Model file for the job. Use its own axes, mm. Face numbers are marked on the shaded views. A direction names the side the tool comes from. Round coordinates to 2 decimals unless told otherwise and drop trailing zeros. Loops run counter-clockwise (first coordinate to the right, second up) from the corner with the lowest first, then second, coordinate; pieces in that order, holes last.
from build123d import *

# Parameters (mm, degrees)
BOSS_EXTRUDE1_DEPTH = 12
SKETCH2_W           = 4
SKETCH2_H           = 1.5
BOSS_EXTRUDE2_DEPTH = 10
CUT_EXTRUDE1_DEPTH  = 2.5
BOSS_EXTRUDE4_DEPTH = 6
SKETCH6_R           = 2.275
BOSS_EXTRUDE5_DEPTH = 3.5


# Read off the part's stored shape, not the designer's step: Boss-Extrude4
with BuildPart() as part:
    # Sketch1 → Boss-Extrude1 (new body)
    with BuildSketch(Plane.XY):
        Polygon((-11.25, 11.3), (11.25, 11.3), (11.25, 9.7), (16.25, 9.7), (16.25, 7.2), (11.25, 7.2), (11.25, -11.3), (-11.25, -11.3), (-11.25, 7.2), (-16.25, 7.2), (-16.25, 9.7), (-11.25, 9.7), align=None)
    extrude(amount=-BOSS_EXTRUDE1_DEPTH)

    # Sketch2 → Boss-Extrude2 (add)
    with BuildSketch(Plane(origin=(11.25, 0, 0), x_dir=(0, 0, -1), z_dir=(1, 0, 0))):
        with Locations((6, -7.05)):
            Rectangle(SKETCH2_W, SKETCH2_H)
    extrude(amount=BOSS_EXTRUDE2_DEPTH)

    # Sketch3 → Cut-Extrude1 (cut)
    with BuildSketch(Plane(origin=(0, 9.7, 0), x_dir=(1, 0, 0), z_dir=(0, 1, 0))):
        with BuildLine():
            Line((-16.25, 6.5), (-14.866025404, 6.5))
            ThreePointArc((-14.866025404, 6.5), (-13, 6), (-14.866025404, 5.5))
            Line((-14.866025404, 5.5), (-16.25, 5.5))
            Line((-16.25, 5.5), (-16.25, 6.5))
        make_face()
        with BuildLine():
            Line((16.25, 6.5), (14.866025404, 6.5))
            ThreePointArc((14.866025404, 6.5), (13, 6), (14.866025404, 5.5))
            Line((14.866025404, 5.5), (16.25, 5.5))
            Line((16.25, 5.5), (16.25, 6.5))
        make_face()
    extrude(amount=-CUT_EXTRUDE1_DEPTH, mode=Mode.SUBTRACT)

    # Boss-Extrude4 outline → Boss-Extrude4 (add)
    with BuildSketch(Plane(origin=(0, 11.3, 0), x_dir=(1, 0, 0), z_dir=(0, 1, 0))):
        with BuildLine():
            Line((-0.204356057, 8.5), (-1.254356051, 8.499996205))
            ThreePointArc((-1.254356051, 8.499996205), (-3.75, 6), (-1.254356051, 3.500003795))
            Line((-1.254356051, 3.500003795), (-0.204356057, 3.5))
            ThreePointArc((-0.204356057, 3.5), (11.25, 6), (-0.204356057, 8.5))
        make_face()
    extrude(amount=BOSS_EXTRUDE4_DEPTH)

    # Sketch6 → Boss-Extrude5 (add)
    with BuildSketch(Plane(origin=(0, 17.3, 0), x_dir=(1, 0, 0), z_dir=(0, 1, 0))):
        with Locations(Location((5.25, 6, 0), (0, 0, 270))):
            Circle(SKETCH6_R)
    extrude(amount=BOSS_EXTRUDE5_DEPTH)


solid = part.part
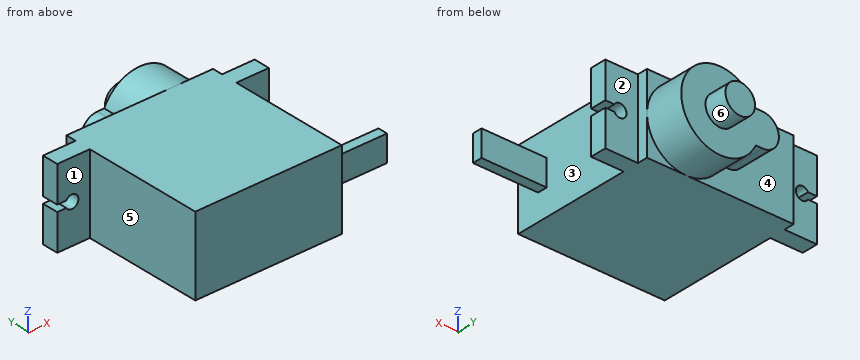
Q1. Pull direction Y, two halves, no side cores. Call the marked faces 1, 2 and 3: pulls with the +Y half, pulls with the -Y half, needs draft (parallel to the pull), parting line crosses it, or undercut.
Q2. Slice it at A-A on x = 14. Give the cut face in (y, z), plus the area to 3 significant figures.
Q3. Slice it at B-B on y = 8.5. Give the cut face in (x, z), plus the area to 3 significant figures.
Q4. Tool access for the marked faces 4, 5 and 6: list every direction of +Z, -Z, +X, -X, +Y, -Y with a clear straight run to the whole face (end or side of a thin tool).
Q5. Slice it at D-D on z = -10. Give the cut face in (x, y), plus the area to 3 significant figures.
Q6. Flat gauge pins, fed straight in: P1, Ø1.5, axis at x = -4, z = -2, coming from the +Y side; P2, Ø3, axis at y = 16.5, z = -3, coming from the +X side; P3, Ø1.5, axis at x = -14.5, z = -6.5, coming from the -Y side. Where does each tip first touch, or does it go through?
Q7. Slice it at C-C on x = -14. Give the cut face in (y, z), plus the area to 3 significant figures.
Q8. Probe line 1 (Z direction, x = -14, y = 9); line 2 (X direction, y = 8.25, z = -6); line 3 (Y direction, x = 5, z = -10). List the from-to ranges inside material, lowest first.
Reply:
1. face 1: pulls with the -Y half
1. face 2: pulls with the +Y half
1. face 3: undercut
2. outline: (-7.8, -8) - (-6.3, -8) - (-6.3, -4) - (-7.8, -4) - close; (7.2, -12) - (9.7, -12) - (9.7, -7) - (7.2, -7) - close; (7.2, -5) - (9.7, -5) - (9.7, 0) - (7.2, 0) - close
2. area: 31.0 mm2
3. outline: (-16.25, -12) - (16.25, -12) - (16.25, -6.5) - (14.87, -6.5) arc R1 cw (long way) to (14.87, -5.5) - (16.25, -5.5) - (16.25, 0) - (-16.25, 0) - (-16.25, -5.5) - (-14.87, -5.5) arc R1 cw (long way) to (-14.87, -6.5) - (-16.25, -6.5) - close
3. area: 381 mm2
4. face 4: -X, +Y
4. face 5: +Z, -Z, -X, -Y
4. face 6: +Y
5. outline: (-16.25, 7.2) - (-11.25, 7.2) - (-11.25, -11.3) - (11.25, -11.3) - (11.25, 7.2) - (16.25, 7.2) - (16.25, 9.7) - (11.25, 9.7) - (11.25, 11.3) - (9.72, 11.3) - (9.72, 17.3) - (0.78, 17.3) - (0.78, 11.3) - (-11.25, 11.3) - (-11.25, 9.7) - (-16.25, 9.7) - close
5. area: 587 mm2
6. P1: stops at y = 11.3
6. P2: stops at x = 11.06
6. P3: stops at y = 7.2
7. outline: (7.2, -12) - (9.7, -12) - (9.7, -7) - (7.2, -7) - close; (7.2, -5) - (9.7, -5) - (9.7, 0) - (7.2, 0) - close
7. area: 25.0 mm2
8. line 1: z = -12 to -7, -5 to 0
8. line 2: x = -13 to 13
8. line 3: y = -11.3 to 17.3
